```python
from build123d import *

# Parameters (mm, degrees)
SKETCH_8_R = 9


with BuildPart() as part:
    # 扫描5: sweep along a curve in space
    with BuildLine() as sweep_5_path:
        Line((0, 62, 0), (0, 60.404917791, 0))
        ThreePointArc((0, 60.404917791, 0), (0, 54.413888405, 1.774623753), (0, 50.355917757, 6.525896926))
        Line((0, 50.355917757, 6.525896926), (0, 35.474103074, 39.950999966))
        ThreePointArc((0, 35.474103074, 39.950999966), (3.221825407, 32.310434451, 47.056716034), (11, 31, 50))
        Line((11, 31, 50), (62, 31, 50))
        ThreePointArc((62, 31, 50), (69.778174593, 29.302292387, 47.261761914), (73, 25.203663643, 40.651070391))
        Line((73, 25.203663643, 40.651070391), (73, 5.796336357, 9.348929609))
        ThreePointArc((73, 5.796336357, 9.348929609), (69.778174593, 1.697707613, 2.738238086), (62, 0, 0))
        Line((62, 0, 0), (43, 0, 0))
    # 草图8 → 扫描5 (sweep)
    with BuildSketch(Plane(origin=(0, 62, 0), x_dir=(1, 0, 0), z_dir=(0, 1, 0))):
        Circle(SKETCH_8_R)
    sweep(path=sweep_5_path.line)


solid = part.part
```
The listing builds one solid part. Answer for the finished solid, in the listing's coordinates (mm). A direction names the side the tool comes from. Give positions to 0.01 mm unless a question says otherwise; leave off trailing zeros. Order: outer loops, then holes, each group sorted by start corner. A loop starts at its lowest first (then second) coordinate and runs counter-clockwise, first axis right, second up.
Item 1: Given pin 1 Ø12 at (x, y) = (14.5, 19.5) entering from -Z; pin 2 Ø1 at (x, z) = (14, 47.5) entering from -Y; pin 3 Ø2 at (x, z) = (13.5, 42.5) entering from +Y; pin 4 Ø5 at (x, z) = (51, 12.5) entering from +Y, each flat-ended and moving along its own axis, determine where each tip first touches the part or whether it passes through.
From the geometry:
pin 1: stops at z = 42.88
pin 2: stops at y = 22.23
pin 3: stops at y = 37.22
pin 4: passes through
Item 2: For a pull along X with two mould halves and no side action, classify faces 3 (the face through (-1.172, 61.191, 8.923)), 4 (the face through (36.857, 27.704, 58.375)), 5 (the face through (43, 0, 0)) as pulls with the +X half, pulls with the -X half, needs draft (parallel to the pull), parting line crosses it, or undercut.
From the geometry:
face 3: parting line crosses it
face 4: undercut
face 5: pulls with the -X half
Item 3: Find the intervals of material crossed by probe 1 along Z at (x, y) = (74, 34); probe 2 along Y at (x, z) = (5, 0.5); probe 3 along X at (y, z) = (24, 33), in increasing order.
From the geometry:
probe 1: z = 37.92 to 54.01
probe 2: y = 45.19 to 62
probe 3: x = 64.52 to 81.48
Item 4: The part is cut by section A-A, the plane x = 18. Give the vertices of the cut face in (y, z), and give its area (3 significant figures).
From the geometry:
outline: circle Ø18 at (31, 50)
area: 254 mm2
Item 5: Which of the six approach directions +Z, -Z, +X, -X, +Y, -Y give full straight-line access (tool end or side, diameter ignored) to faces 1 (the face through (52.4, 8.7, -2.3)), 2 (the face through (-1.172, 50.963, 27.102))?
From the geometry:
face 1: -X
face 2: none
